Could you check a few things on this model? Use its own coordinates, in mm. A direction names the side the tool comes from. Coordinates: 2 decimals unless noted, no trailing zeros. Loops run counter-clockwise (first coordinate to the right, second up) from the corner with the lowest first, then second, coordinate; pieces in that order, holes last. Notation, with made-up numbers: (77, 34) -> (127, 34) arc R12 cw to (127, 53) -> close; hole circle Ø10 at (57, 36). An arc over 180 degrees is marked (long way). One line per question, with ' | ' between items.
Autodesk Inventor part; units mm, degrees
ref_plane "YZ Plane" through (0, 0, 0) normal (1, 0, 0) x (0, 1, 0)
ref_plane "XZ Plane" through (0, 0, 0) normal (0, 1, 0) x (-1, 0, 0)
ref_plane "XY Plane" through (0, 0, 0) normal (0, 0, 1) x (1, 0, 0)
sketch "Sketch1" plane through (0, 0, 0) normal (1, 0, 0) x (0, 1, 0)
  line L0 (12.0648, 10.4185) -> (22.0648, 10.4185)
  line L1 (22.0648, 10.4185) -> (22.0648, -17.5815)
  line L2 (22.0648, -17.5815) -> (12.0648, -17.5815)
  line L3 (12.0648, -17.5815) -> (12.0648, 10.4185)
  point P0 (0, 0)
  dimension "d0" = 28
  dimension "d1" = 10
extrude "Extrusion1" add sketch "Sketch1" along normal blind 10
sketch "Sketch2" plane through (0, 12.0648, -17.5815) normal (0, -1, 0) x (1, 0, 0)
  line L0 (0, 28) -> (10, 28)
  line L1 (0, 0) -> (10, 0)
  line L2 (0, 28) -> (2, 28)
  line L3 (2, 28) -> (2, 0)
  line L4 (2, 0) -> (0, 0)
  line L5 (0, 0) -> (0, 28)
  point P0 (0, 17.5815)
  dimension "d4" = 2
extrude "Extrusion2" add sketch "Sketch2" along normal blind 1.7
sketch "Sketch3" plane through (10, 12.0648, -17.5815) normal (0, -1, 0) x (1, 0, 0)
  circle A0 centre (-4, 8) radius 0.8
  circle A1 centre (-4, 17) radius 0.8
  line L0 (-8, 0) -> (0, 0)
  line L1 (-8, 0) -> (-8, 28)
  point P0 (-10, 17.5815)
  dimension "d7" = 1.6
  dimension "d8" = 1.6
  dimension "d9" = 8
  dimension "d10" = 9
  dimension "d11" = 4
  dimension "d12" = 4
extrude "Extrusion3" cut sketch "Sketch3" against normal through all
sketch "Sketch4" plane through (10, 0, 0) normal (1, 0, 0) x (0, 0, -1)
  circle A0 centre (-5.4185, 17.0648) radius 1.05
  circle A1 centre (3.5815, 17.0648) radius 1.05
  circle A2 centre (12.5815, 17.0648) radius 1.05
  line L0 (17.5815, 22.0648) -> (-10.4185, 22.0648)
  line L1 (17.5815, 12.0648) -> (17.5815, 22.0648)
  point P0 (0, 0)
  dimension "d15" = 2.1
  dimension "d16" = 2.1
  dimension "d17" = 2.1
  dimension "d18" = 5
  dimension "d19" = 5
  dimension "d20" = 5
  dimension "d21" = 5
  dimension "d22" = 9
  dimension "d23" = 9
extrude "Extrusion4" cut sketch "Sketch4" against normal through all
sketch "Sketch5" plane through (10, 0, 0) normal (1, 0, 0) x (0, 0, -1)
  circle A0 centre (-5.4185, 17.0648) radius 1.05
  circle A1 centre (-5.4185, 17.0648) radius 2
  circle A2 centre (3.5815, 17.0648) radius 1.05
  circle A3 centre (3.5815, 17.0648) radius 2
  circle A4 centre (12.5815, 17.0648) radius 1.05
  circle A5 centre (12.5815, 17.0648) radius 2
  point P0 (0, 0)
  dimension "d26" = 4
  dimension "d27" = 4
  dimension "d28" = 4
extrude "Extrusion5" cut sketch "Sketch5" against normal blind 2.5
chamfer "Chamfer1" distance 0.9 angle 45 3 edges at (7.5, 17.0648, 6.4685) (7.5, 17.0648, -2.5315) (7.5, 17.0648, -11.5315)
sketch "Sketch6" plane through (10, 22.0648, -17.5815) normal (0, 0, -1) x (-1, 0, 0)
  line L0 (0, 0) -> (0, -10)
  line L1 (0, -10) -> (0, 0)
  line L2 (0, 0) -> (10, 0)
  line L3 (8, -11.7) -> (10, -11.7)
  line L4 (10, 0) -> (10, -11.7)
  line L5 (8, -11.7) -> (8, -10)
  line L6 (8, -10) -> (0, -10)
  point P0 (10, -22.0648)
extrude "Extrusion6" add sketch "Sketch6" along normal blind 9
sketch "Sketch7" plane through (2, 12.0648, 10.4185) normal (0, -1, 0) x (1, 0, 0)
  circle A0 centre (4, -29) radius 0.8
  line L0 (0, 0) -> (0, -37)
  line L1 (8, -37) -> (0, -37)
  point P0 (-2, -10.4185)
  dimension "d39" = 1.6
  dimension "d40" = 4
  dimension "d41" = 8
extrude "Extrusion7" cut sketch "Sketch7" against normal through all
properties part number "probe_mount"
Q1. Imagine slicing it at B-B on y = 20.5. Write out the boundary of the cut face in (x, z).
Values follow:
outline: (0, -26.58) -> (10, -26.58) -> (10, 10.42) -> (0, 10.42) -> close; hole circle Ø1.6 at (6, -18.58); hole circle Ø1.6 at (6, -9.58); hole circle Ø1.6 at (6, -0.58)
Q2. Imagine slicing it at C-C on x = 1.5. Write out the boundary of the cut face in (y, z), plus the area to 3 significant figures.
Values follow:
outline: (10.36, -26.58) -> (22.06, -26.58) -> (22.06, 10.42) -> (10.36, 10.42) -> close; hole circle Ø2.1 at (17.06, -12.58); hole circle Ø2.1 at (17.06, -3.58); hole circle Ø2.1 at (17.06, 5.42) | area: 423 mm2
Q3. For pin 1 (3 mm diameter, centred on y = 17, z = -4, fed in from +X); pin 2 (2.5 mm diameter, centred on y = 17.06, z = -3.58, fed in from +X) (3 decimals); pin 3 (2.5 mm diameter, centred on x = 6, z = -0.58, fed in from -Y), each with a flat end and sliding along its axis, tell me the tip position at first contact or that it passes through.
Values follow:
pin 1: stops at x = 7.47 | pin 2: stops at x = 6.805 | pin 3: stops at y = 12.06
Q4. We'd pull the mould along Y, two halves only. Please class faces 4 (the face through (6, 12.065, -8)), 5 (the face through (5.2, 16.99, -0.55)), 6 (the face through (3.35, 16.04, -3.35)): released by +Y, released by -Y, zero draft, split by the parting line, or undercut.
Values follow:
face 4: released by -Y | face 5: zero draft | face 6: undercut
Q5. Imagine slicing it at A-A on x = 6. Write out the boundary of the cut face in (y, z), plus the area to 3 significant figures.
Values follow:
outline: (12.06, -26.58) -> (22.06, -26.58) -> (22.06, -19.38) -> (12.06, -19.38) -> close; (12.06, -17.78) -> (22.06, -17.78) -> (22.06, -10.38) -> (12.06, -10.38) -> close; (12.06, -8.78) -> (22.06, -8.78) -> (22.06, -1.38) -> (12.06, -1.38) -> close; (12.06, 0.22) -> (22.06, 0.22) -> (22.06, 10.42) -> (12.06, 10.42) -> close; hole circle Ø2.1 at (17.06, -12.58); hole circle Ø2.1 at (17.06, -3.58); hole circle Ø2.1 at (17.06, 5.42) | area: 312 mm2
Q6. For faces 1 (the face through (8.77, 15.11, 5.85)), 2 (the face through (2, 11, -8)), 3 (the face through (5.41, 16.99, -9.04)), which set-ups out of +Z, -Z, +X, -X, +Y, -Y let a thin tool reach every point of the face, with its end or its side?
Values follow:
face 1: +X | face 2: +Z, -Z, +X, -Y | face 3: +Y, -Y
Q7. Please list where these lines run through material, in increasing order: L1, parallel to Z at x = 9.5, y = 17.25; L2, parallel to Z at x = 6, y = 18.25; L3, parallel to Y at x = 8, z = -7.5. Write a range as [from, to].
Values follow:
L1: z = [-26.58, -14.57], [-10.59, -5.57], [-1.59, 3.43], [7.41, 10.42] | L2: z = [-26.58, -19.38], [-17.78, -10.38], [-8.78, -1.38], [0.22, 10.42] | L3: y = [12.06, 22.06]
